Here's how the part is built. I have some questions about the finished solid (model axes, mm). Round coordinates to 2 decimals unless told otherwise and drop trailing zeros. Loops run counter-clockwise (first coordinate to the right, second up) from the corner with the lowest first, then second, coordinate; pieces in that order, holes last. Notation, with made-up numbers: M 58,55.25 L 75,55.25 A25 ccw 75,69.25 Z; hole C 64.25,65 d6. An arc over 180 degrees is marked long. Answer as a JSON object with one key per item and string values.
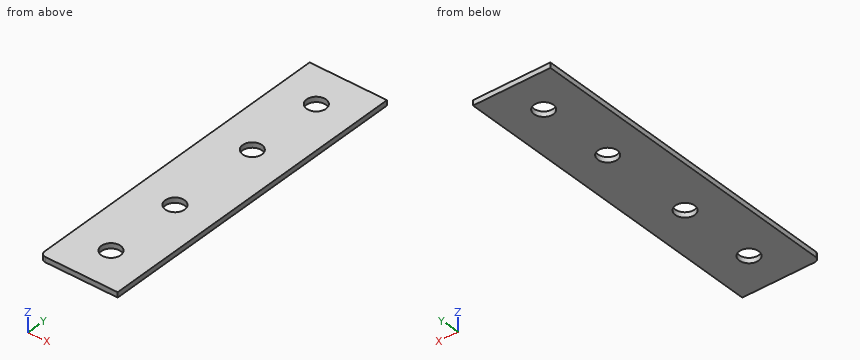
Autodesk Inventor part; units mm, degrees
ref_plane "YZ Plane" through (0, 0, 0) normal (1, 0, 0) x (0, 1, 0)
ref_plane "XZ Plane" through (0, 0, 0) normal (0, 1, 0) x (-1, 0, 0)
ref_plane "XY Plane" through (0, 0, 0) normal (0, 0, 1) x (1, 0, 0)
sketch "Sketch1" plane through (0, 0, 0) normal (0, 0, 1) x (1, 0, 0)
  arc A0 (10.4999, 13) -> (8.4999, 15) centre (8.4999, 13) ccw
  arc A1 (-19.5, -109.2599) -> (-17.5, -111.2599) centre (-17.5, -109.2599) ccw
  line L0 (10.4999, 15) -> (-19.5, 15)
  line L1 (-19.5, 15) -> (-19.5, -111.2599)
  line L2 (-19.5, -111.2599) -> (10.4999, -111.2599)
  line L3 (10.4999, -111.2599) -> (10.4999, 15)
  line L4 (-4.5, -111.2599) -> (-4.5, 15) construction
  circle A2 centre (-4.5, 0) radius 3.75
  circle A3 centre (-4.5, -30) radius 3.75
  circle A4 centre (-4.5, -66.2599) radius 3.75
  circle A5 centre (-4.5, -96.2599) radius 3.75
  point P0 (0, 0)
  dimension "d0" = 29.9999
  dimension "d1" = 126.2599
  dimension "d2" = 7.5
  dimension "d3" = 15
  dimension "d4" = 15
  dimension "d5" = 30
  dimension "d6" = 30
extrude "Plate1" add sketch "Sketch1" along normal blind 2 contours L3 L2 A1 L1 L0 A0 | A0 L0 L3
equation "\"d4\" = d3"
equation "\"d6\" = d5"
equation "\"BendRadius\" = Thickness"
equation "\"BendReliefWidth\" = Thickness"
equation "\"BendReliefDepth\" = 0.5 * Thickness"
equation "\"CornerReliefSize\" = 4 * Thickness"
equation "\"MinimumRemnant\" = 2 * Thickness"
equation "\"TransitionRadius\" = BendRadius"
equation "\"JacobiRadiusSize\" = BendRadius"
equation "\"GapSize\" = Thickness"
equation "\"d7\" = BendRadius"
properties part number "gabarito-suporte-motor-lateral" material "Wood (Oak)"
Item 1: If I drill on L1, parallel to Y at x = -4.5, z = 0.45; L2, parallel to Y at x = -6.5, z = 1.65; L3, parallel to X at y = -68, z = 1.25, over which ranges is the centre line in solid material (lowest first)? Write a range as from..to.
Solution:
{"L1": "y = -111.26..-100.01, -92.51..-70.01, -62.51..-33.75, -26.25..-3.75, 3.75..15", "L2": "y = -111.26..-99.43, -93.09..-69.43, -63.09..-33.17, -26.83..-3.17, 3.17..15", "L3": "x = -19.5..-7.82, -1.18..10.5"}
Item 2: For P1, Ø7, axis at x = -4.5, y = 0, coming from the -Z side, with a flat end and sliding along its axis, tell me the tip position at first contact or that it passes through.
Solution:
{"P1": "passes through"}
Item 3: I want a section at A-A on y = 0. List the corners of the cut face in (x, z) for me.
Solution:
{"outline": "M -19.5,0 L -8.25,0 L -8.25,2 L -19.5,2 Z; M -0.75,0 L 10.5,0 L 10.5,2 L -0.75,2 Z"}
Item 4: I want a section at C-C on z = 1.65. List the corners of the cut face in (x, y) for me, plus the area to 3 significant figures.
Solution:
{"outline": "M -19.5,-109.26 A2 ccw -17.5,-111.26 L 10.5,-111.26 L 10.5,15 L -19.5,15 Z; hole C -4.5,-96.26 d7.5; hole C -4.5,-66.26 d7.5; hole C -4.5,-30 d7.5; hole C -4.5,0 d7.5", "area": "3,610 mm2"}
Item 5: I want a section at B-B on x = -4.5. List the corners of the cut face in (y, z) for me.
Solution:
{"outline": "M -111.26,0 L -100.01,0 L -100.01,2 L -111.26,2 Z; M -92.51,0 L -70.01,0 L -70.01,2 L -92.51,2 Z; M -62.51,0 L -33.75,0 L -33.75,2 L -62.51,2 Z; M -26.25,0 L -3.75,0 L -3.75,2 L -26.25,2 Z; M 3.75,0 L 15,0 L 15,2 L 3.75,2 Z"}
